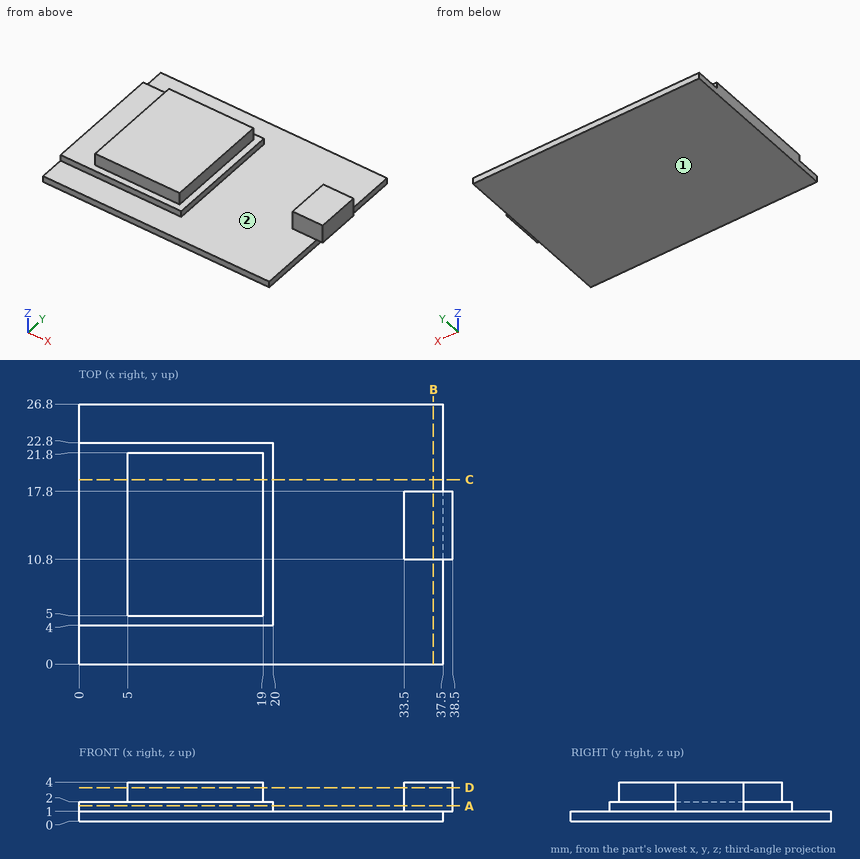
For this review, use the dimensioned drawing (mm, ordinates from the lowest corner) and the shaded views. Give positions to 0.01 mm unless a question says otherwise; leave off trailing zeros. Write each loop counter-clockwise with the first axis right and the second up, starting at its lowest first coordinate (ties: lowest second). Pieces come first, ordered by that corner, then holes. Notation, with made-up numbers: M 49,51 L 104,51 A14 cw 104,72 Z; hole C 81,3.25 d1. An arc over 180 degrees is marked long. Answer as a JSON object with one key per item and string values. Group by question number.
Item 1: Consider section C-C on y = 19. Write out the cut boundary in (x, z), plus the area to 3 significant figures.
Item 2: Consider section D-D on z = 3.45. Write out the cut boundary in (x, y).
Item 3: For pin 1 Ø2 at (x, z) = (11.5, 2.5) entering from -Y; pin 2 Ø0.6 at (x, z) = (10.5, 3.5) entering from +Y; pin 3 Ø1.5 at (x, z) = (36.5, 3) entering from +Y, all flat-tipped, find the tip position at first contact; note any pin that passes through.
Item 4: Consider section B-B on x = 36.5. Write out the cut boundary in (y, z).
Item 5: Consider section A-A on z = 1.55. Write out the cut boundary in (x, y), plus the area to 3 significant figures.
Item 6: Draft analysis for pull direction X (two halves, no side actions). For the marked faces 1 and 2, state which applies: +X half, -X half, draft (parallel to the pull), parting line (faces both ways), or undercut.
Item 7: For probe 1 along X at (y, z) = (16.75, 2.65); probe 2 along X at (y, z) = (13, 1.35); probe 3 along X at (y, z) = (20.5, 3.8), list the stretches that pass through material, from the lowest coordinate up. Write a range as [from, to].
Check result:
{
 "1": {"outline": "M 0,0 L 37.5,0 L 37.5,1 L 20,1 L 20,2 L 19,2 L 19,4 L 5,4 L 5,2 L 0,2 Z", "area": "85.5 mm^2"},
 "2": {"outline": "M 5,5 L 19,5 L 19,21.8 L 5,21.8 Z; M 33.5,10.8 L 38.5,10.8 L 38.5,17.8 L 33.5,17.8 Z"},
 "3": {"pin 1": "stops at y = 4", "pin 2": "stops at y = 21.8", "pin 3": "stops at y = 17.8"},
 "4": {"outline": "M 0,0 L 26.8,0 L 26.8,1 L 17.8,1 L 17.8,4 L 10.8,4 L 10.8,1 L 0,1 Z"},
 "5": {"outline": "M 0,4 L 20,4 L 20,22.8 L 0,22.8 Z; M 33.5,10.8 L 38.5,10.8 L 38.5,17.8 L 33.5,17.8 Z", "area": "411 mm^2"},
 "6": {"face 1": "draft", "face 2": "undercut"},
 "7": {"probe 1": "x = [5, 19], [33.5, 38.5]", "probe 2": "x = [0, 20], [33.5, 38.5]", "probe 3": "x = [5, 19]"}
}
